Autodesk Inventor part; units mm, degrees
ref_plane "Work Plane1" through (0, 0, -15) normal (0, 0, 1) x (1, 0, 0)
ref_plane "YZ Plane" through (0, 0, 0) normal (1, 0, 0) x (0, 1, 0)
ref_plane "XZ Plane" through (0, 0, 0) normal (0, 1, 0) x (-1, 0, 0)
sketch "Sketch1" plane through (0, 0, 0) normal (0, 0, 1) x (1, 0, 0)
  line L0 (0, 0) -> (25, 0)
  line L1 (25, 0) -> (25, 40)
  line L2 (25, 40) -> (0, 40)
  line L3 (0, 40) -> (0, 0)
  dimension "d1" = 25
  dimension "d2" = 40
  dimension "d3" = 25
extrude "Extrusion1" add sketch "Sketch1" against normal blind 30
sketch "Sketch2" plane through (25, 0, 0) normal (1, 0, 0) x (0, 0, -1)
  line L0 (0, 0) -> (30, 0)
  circle A0 centre (15, 6.56) radius 2.46
extrude "Extrusion2" cut sketch "Sketch2" against normal blind 30
sketch "Sketch3" plane through (0, 0, 0) normal (-1, 0, 0) x (0, 0, 1)
  line L0 (0, 0) -> (-30, 0)
  line L1 (-25.05, 0) -> (-4.95, 0)
  line L2 (-4.95, 0) -> (-4.95, 33.12)
  line L3 (-4.95, 33.12) -> (-25.05, 33.12)
  line L4 (-25.05, 33.12) -> (-25.05, 0)
  dimension "d11" = 20.1
extrude "Extrusion3" cut sketch "Sketch3" against normal blind 20
sketch "Sketch4" plane through (0, 0, 0) normal (0, -1, 0) x (1, 0, 0)
  line L0 (20, -4.95) -> (20, -25.05)
  line L1 (20, -15) -> (25, -15)
  line L2 (25, 0) -> (25, -30)
  line L3 (20, -8.025) -> (25, -8.025)
  line L4 (25, -8.025) -> (25, -21.975)
  line L5 (25, -21.975) -> (20, -21.975)
  line L6 (20, -21.975) -> (20, -8.025)
  line L7 (20, -8.025) -> (25, -21.975) construction
  line L8 (25, -8.025) -> (20, -21.975) construction
  line L9 (25, -12.54) -> (25, -17.46)
  point P0 (0, 0)
  point P1 (22.5, -15)
  dimension "d14" = 13.95
extrude "Extrusion4" add sketch "Sketch4" along normal blind 15
sketch "Sketch5" plane through (20, 0, 0) normal (-1, 0, 0) x (0, 0, 1)
  circle A0 centre (-15, 6.56) radius 2.46
  circle A1 centre (-15, 6.56) radius 4.7025
  circle A2 centre (-15, 6.56) radius 2.46
  circle A3 centre (-15, 6.56) radius 2.46
  point P0 (0, 0)
  dimension "d17" = 9.405
extrude "Extrusion5" cut sketch "Sketch5" against normal blind 2.1
sketch "Sketch6" plane through (25, 0, 0) normal (1, 0, 0) x (0, 0, -1)
  circle A0 centre (15, 6.56) radius 4.7025
  line L0 (15, 6.56) -> (15, 23.56)
  circle A1 centre (15, 23.56) radius 2.46
  point P0 (0, 0)
  dimension "d20" = 17
  dimension "d21" = 4.92
extrude "Extrusion6" cut sketch "Sketch6" against normal blind 10 contours A1
sketch "Sketch7" plane through (20, 0, 0) normal (-1, 0, 0) x (0, 0, 1)
  circle A0 centre (-15, 23.56) radius 2.46
  circle A1 centre (-15, 23.56) radius 4.7025
  point P0 (0, 0)
  dimension "d24" = 9.405
extrude "Extrusion7" cut sketch "Sketch7" against normal blind 2.1
sketch "Sketch9" plane through (25, 0, 0) normal (1, 0, 0) x (0, 0, -1)
  circle A0 centre (15, 6.56) radius 2.46
  circle A1 centre (15, 6.56) radius 2.46
  circle A2 centre (15, 23.56) radius 2.46
  circle A3 centre (15, 23.56) radius 2.46
  line L0 (30, 40) -> (30, 0)
  line L1 (30, 0) -> (30, 40)
  line L2 (30, 40) -> (0, 40)
  line L3 (0, 40) -> (0, 0)
  line L4 (0, 0) -> (8.025, 0)
  line L5 (21.975, 0) -> (21.975, -15)
  line L6 (21.975, -15) -> (8.025, -15)
  line L7 (8.025, -15) -> (8.025, 0)
  line L8 (0, 0) -> (8.025, 0)
  line L9 (21.975, 0) -> (30, 0)
extrude "Extrusion8" add sketch "Sketch9" along normal blind 5
sketch "Sketch10" plane through (0, 40, 0) normal (0, 1, 0) x (1, 0, 0)
  line L0 (0, 30) -> (30, 30)
  line L1 (30, 0) -> (0, 0)
  line L2 (0, 30) -> (30, 30)
  line L3 (30, 30) -> (30, 0)
  line L4 (30, 0) -> (0, 0)
  line L5 (0, 0) -> (0, 30)
extrude "Extrusion9" add sketch "Sketch10" along normal blind 30
sketch "Sketch12" plane through (30, 0, 0) normal (1, 0, 0) x (0, 0, -1)
  circle A0 centre (15, 6.56) radius 2.46
  line L0 (15, 6.56) -> (15, 15.06)
  circle A1 centre (15, 15.06) radius 2.525
  point P0 (0, 0)
  dimension "d31" = 8.5
  dimension "d33" = 5.05
extrude "Extrusion10" cut sketch "Sketch12" against normal blind 30 contours A1
sketch "Sketch15" plane through (0, 0, -25.05) normal (-1, 0, 0) x (0, 0, 1)
  line L0 (0, 33.12) -> (20.1, 33.12)
  line L1 (20.1, 33.12) -> (20.1, 0)
  line L2 (0, 33.12) -> (20.1, 33.12)
  line L3 (20.1, 33.12) -> (20.1, 31.1)
  line L4 (20.1, 31.1) -> (0, 31.1)
  line L5 (0, 31.1) -> (0, 33.12)
  point P0 (25.05, 0)
  dimension "d57" = 2.02
extrude "Extrusion13" add sketch "Sketch15" against normal blind 20
sketch "Sketch17" plane through (0, 0, 0) normal (0, 0, 1) x (1, 0, 0)
  line L0 (0, 70) -> (30, 70)
  line L1 (30, 70) -> (50.0622, 90.0622)
  line L2 (30, 70) -> (80, 70) construction
  line L3 (11.9522, 97.2454) -> (0, 85.2932)
  line L4 (0, 70) -> (0, 85.2932)
  line L5 (0, 70) -> (0, 0)
  line L6 (0, 70) -> (30, 70)
  line L7 (10.923, 112.2849) -> (0, 120.567)
  line L8 (50.0622, 105.3553) -> (50.0622, 120.567)
  line L9 (50.0622, 105.3553) -> (50.0622, 90.0622)
  arc A0 (11.9522, 97.2454) -> (10.923, 112.2849) centre (4.8811, 104.3165) ccw
  line L10 (0, 156.567) -> (30, 156.567)
  line L11 (30, 156.567) -> (50.0622, 120.567)
  line L12 (5, 154.567) -> (0, 156.567)
  line L13 (5, 122.567) -> (0, 120.567)
  line L14 (5, 122.567) -> (10, 138.567)
  line L15 (10, 138.567) -> (5, 154.567)
  dimension "d61" = 45
  dimension "d62" = 32.0271
  dimension "d72" = 10
extrude "Extrusion14" add sketch "Sketch17" against normal blind 30
sketch "Sketch23" plane through (0, 0, 0) normal (0, 0, 1) x (1, 0, 0)
  line L0 (50.0622, 90.0622) -> (30, 70)
  line L1 (30, 70) -> (50.0622, 90.0622)
  line L2 (50.0622, 120.567) -> (50.0622, 90.0622)
  line L3 (50.0622, 90.0622) -> (50.0622, 120.567)
  line L4 (30, 156.567) -> (50.0622, 120.567)
  line L5 (50.0622, 120.567) -> (30, 156.567)
  line L6 (0, 156.567) -> (30, 156.567)
  line L7 (30, 156.567) -> (0, 156.567)
  line L8 (5, 154.567) -> (0, 156.567)
  line L9 (0, 156.567) -> (5, 154.567)
  line L10 (10, 138.567) -> (5, 154.567)
  line L11 (5, 154.567) -> (10, 138.567)
  line L12 (5, 122.567) -> (10, 138.567)
  line L13 (10, 138.567) -> (5, 122.567)
  line L14 (0, 120.567) -> (5, 122.567)
  line L15 (5, 122.567) -> (0, 120.567)
  line L16 (10.923, 112.2849) -> (0, 120.567)
  line L17 (0, 120.567) -> (10.923, 112.2849)
  line L18 (0, 85.2932) -> (11.9522, 97.2454)
  line L19 (11.9522, 97.2454) -> (0, 85.2932)
  line L20 (0, 85.2932) -> (0, 55.2932)
  line L21 (0, 0) -> (0, 85.2932)
  line L22 (0, 55.2932) -> (30, 55.2932)
  line L23 (30, 0) -> (30, 70)
  line L24 (30, 55.2932) -> (30, 70)
  arc A0 (11.9522, 97.2454) -> (10.923, 112.2849) centre (4.8811, 104.3165) ccw
  dimension "d97" = 30
extrude "Extrusion15" add sketch "Sketch23" along normal blind 45
ref_plane "Work Plane1" through (0, 0, -15) normal (0, 0, 1) x (1, 0, 0)
mirror "Mirror1" about plane through (0, 0, -15) normal (0, 0, 1) of "Extrusion15"
properties part number "rec_c_32mm_x_120mm"
Verification items for the finished model (mm, model axes). A direction names the side the tool comes from. Round coordinates to 2 decimals unless told otherwise and drop trailing zeros. Write each loop counter-clockwise with the first axis right and the second up, starting at its lowest first coordinate (ties: lowest second). Pieces come first, ordered by that corner, then holes.
1. Section check D-D on y = 34. Enter the section's corners in (x, z).
2. Scan lines: L1, parallel to Y at x = 26, z = -15 (3 decimals); L2, parallel to Z at x = 21, y = 6; L3, parallel to Z at x = 16, y = 5. Record each from-to range of solid material in increasing order.
3. Draft check along Z on faces 4 (the flat face through (20, 8, -20)), 5 (the flat face through (15, 28, 0)), 6 (the flat face through (2.465, 155.581, -14.16)), 7 (the flat face through (22.1, 21.5, -13)). Enter one of: +Z half, -Z half, draft (parallel to the pull), parting line (faces both ways), or undercut.
4. Access from +Z, -Z, +X, -X, +Y, -Y to the whole of each face (thin tool, end or side, straight path). Record for faces 1 (the flat face through (15, 28, -30)), 2 (the flat face through (10, 31.1, -15)), 3 (the flat face through (7.535, 130.679, -14.16)).
5. Section check A-A on y = 15.06. Enter the section's corners in (x, z) (3 decimals), plus the area to 4 significant figures.
6. Section check B-B on z = -46. Enter the section's corners in (x, y), plus the area to 3 significant figures.
7. Gauge pin test, flat ends, axial feed: P1, Ø5.5, axis at y = 23.56, z = -15, coming from the +X side; P2, Ø9, axis at x = 14, z = -2, coming from the -Y side; P3, Ø10, axis at y = -1, z = -17, coming from the -X side; P4, Ø4, axis at y = 6.56, z = -15, coming from the +X side. Record the tip position at first contact, or that the pin passes through.
8. Section check C-C on z = -15. State how many separate pieces and enclosed holes the cut face has, plus the area to 3 significant figures.
Answer:
1. outline: (0, -30) - (30, -30) - (30, 0) - (0, 0) - close
2. L1: y = -15 to 4.1, 9.02 to 12.535, 17.585 to 21.1, 26.02 to 156.567
2. L2: z = -30 to -19.67, -10.33 to 0
2. L3: z = -30 to -25.05, -4.95 to 0
3. face 4: undercut
3. face 5: +Z half
3. face 6: draft
3. face 7: undercut
4. face 1: -Z, +X, -X, -Y
4. face 2: -X, -Y
4. face 3: +Z, -Z, -X
5. outline: (0, -30) - (30, -30) - (30, -17.525) - (20, -17.525) - (20, -25.05) - (0, -25.05) - close; (0, -4.95) - (20, -4.95) - (20, -12.475) - (30, -12.475) - (30, 0) - (0, 0) - close
5. area: 447.5 mm2
6. outline: (0, 55.29) - (30, 55.29) - (30, 70) - (50.06, 90.06) - (50.06, 120.57) - (30, 156.57) - (0, 156.57) - (5, 154.57) - (10, 138.57) - (5, 122.57) - (0, 120.57) - (10.92, 112.28) arc R10 cw to (11.95, 97.25) - (0, 85.29) - close
6. area: 3,640 mm2
7. P1: stops at x = 30
7. P2: stops at y = 0
7. P3: stops at x = 20
7. P4: passes through
8. separate pieces: 4
8. enclosed holes: 0
8. area: 4,660 mm2
